from build123d import *

# Parameters (mm, degrees)
SKETCH_R      = 11.5
SKETCH_R_2    = 7.5
PAD_DEPTH     = 4
SKETCH001_R   = 12.25
SKETCH001_R_2 = 11.5
PAD001_DEPTH  = 4
SKETCH002_R   = 11.5
SKETCH002_R_2 = 8.5
PAD002_DEPTH  = 1


with BuildPart() as part:
    # Sketch → Pad (new body)
    with BuildSketch(Plane.XY):
        Circle(SKETCH_R)
        Circle(SKETCH_R_2, mode=Mode.SUBTRACT)
    extrude(amount=PAD_DEPTH)

    # Sketch001 (on Face3 of Pad) → Pad001 (join)
    with BuildSketch(Plane(origin=(0, 0, 1), x_dir=(1, 0, 0), z_dir=(0, 0, -1))):
        Circle(SKETCH001_R)
        Circle(SKETCH001_R_2, mode=Mode.SUBTRACT)
    extrude(amount=-PAD001_DEPTH)

    # Sketch002 (on Face6 of Pad001) → Pad002 (join)
    with BuildSketch(Plane.XY.offset(4)):
        Circle(SKETCH002_R)
        Circle(SKETCH002_R_2, mode=Mode.SUBTRACT)
    extrude(amount=PAD002_DEPTH)


solid = part.part
Geometry: final body of the model. Coordinates: model frame, mm. A direction names the side the tool comes from. Round coordinates to 2 decimals unless told otherwise and drop trailing zeros. Loops run counter-clockwise (first coordinate to the right, second up) from the corner with the lowest first, then second, coordinate; pieces in that order, holes last.
Q1. Access query for faces 4 (the flat face through (-11, 4, 1)), 5 (the cylindrical face through (4.57, 7.167, 4.493)), 6 (the flat face through (-8.3, -2.6, 5)). Directions: +Z, -Z, +X, -X, +Y, -Y. A direction counts if a zero-diameter tool reaches every point of the face in a straight line with its end or side. Return the directions, or none.
Q2. Section A-A on x = 0. Return loops of the section in (y, z).
Q3. Pin query (flat end, axial travel): P1, Ø12, axis at x = 0, y = 0, coming from the -Z side; P2, Ø1.5, axis at x = -8, z = 3, coming from the -Y side; P3, Ø13.5, axis at x = -0.5, y = 1, coming from the +Z side; P4, Ø3, axis at x = -4, z = 2, coming from the -Y side. Return the tip coordinate at first contact, or that it passes through.
Q4. Material intervals for L1, parallel to Y at x = 0, z = 2; L2, parallel to Y at x = 0, z = 4.5; L3, parallel to X at y = 1.75, z = 2.85, sorted ascending.
Q5. Section C-C on z = 1.55. Return loops of the section in (x, y), plus the area to 3 significant figures.
Q6. Pull-direction query (Y, two-part tool) for faces 1 (the cylindrical face through (-1.5, 11.4, 0.5)), 2 (the flat face through (8, 0, 0)), 3 (the cylindrical face through (-7.493, 0.33, 1.972)); classes: released by +Y, released by -Y, zero draft, split by the parting line, or undercut.
Q7. Section D-D on x = -8. Return loops of the section in (y, z).
Evaluation:
1. face 4: -Z
1. face 5: +Z
1. face 6: +Z, +X, -X, +Y, -Y
2. outline: (-12.25, 1) - (-11.5, 1) - (-11.5, 0) - (-7.5, 0) - (-7.5, 4) - (-8.5, 4) - (-8.5, 5) - (-12.25, 5) - close; (7.5, 0) - (11.5, 0) - (11.5, 1) - (12.25, 1) - (12.25, 5) - (8.5, 5) - (8.5, 4) - (7.5, 4) - close
3. P1: passes through
3. P2: stops at y = -9.87
3. P3: stops at z = 4
3. P4: stops at y = -11.99
4. L1: y = -12.25 to -7.5, 7.5 to 12.25
4. L2: y = -12.25 to -8.5, 8.5 to 12.25
4. L3: x = -12.12 to -7.29, 7.29 to 12.12
5. outline: circle Ø24.5 at (0, 0); hole circle Ø15 at (0, 0)
5. area: 295 mm2
6. face 1: split by the parting line
6. face 2: zero draft
6. face 3: undercut
7. outline: (-9.28, 1) - (-8.26, 1) - (-8.26, 0) - (8.26, 0) - (8.26, 1) - (9.28, 1) - (9.28, 5) - (2.87, 5) - (2.87, 4) - (-2.87, 4) - (-2.87, 5) - (-9.28, 5) - close
